Geometry: final body of the model. Coordinates: model frame, mm. Face numbers are marked on the shaded views. A direction names the side the tool comes from. Give positions to 0.01 mm unless a question says otherwise; leave off trailing zeros. Write each loop counter-clockwise with the first axis right and the second up, starting at its lowest first coordinate (ties: lowest second). Pieces come first, ordered by that corner, then holes.
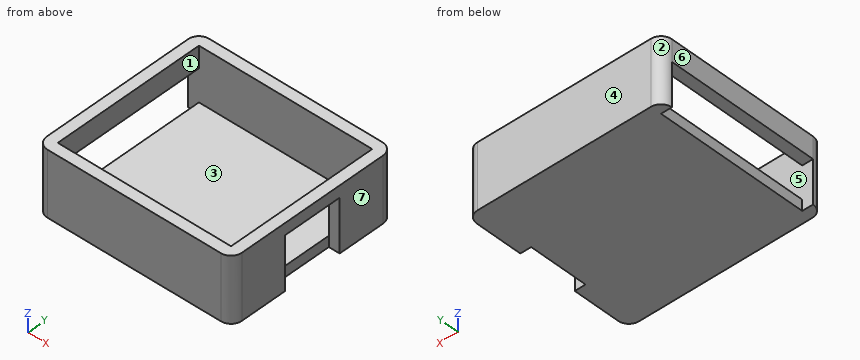
from build123d import *

# Parameters (mm, degrees)
F1_DEPTH = 19.05
F2_T     = 3.175
F3_W     = 17.145
F3_H     = 15.621
F4_DEPTH = 3.175
F5_W     = 44.45
F5_H     = 12.7
F6_DEPTH = 3.175


# Not quite as in the source:
# - a shell that OpenCascade refuses in one call is made with other operations: the cavity is built on its own and cut out


with BuildPart() as f1:
    # F0 (on Top) → F1 (new body)
    with BuildSketch(Plane.XY):
        with BuildLine():
            Line((-25.4, -25.4), (25.4, -25.4))
            ThreePointArc((25.4, -25.4), (27.6450640303, -24.4700640303), (28.575, -22.225))
            Line((28.575, -22.225), (28.575, 22.225))
            ThreePointArc((28.575, 22.225), (27.6450640303, 24.4700640303), (25.4, 25.4))
            Line((25.4, 25.4), (-25.4, 25.4))
            ThreePointArc((-25.4, 25.4), (-27.6450640303, 24.4700640303), (-28.575, 22.225))
            Line((-28.575, 22.225), (-28.575, -22.225))
            ThreePointArc((-28.575, -22.225), (-27.6450640303, -24.4700640303), (-25.4, -25.4))
        make_face()
    extrude(amount=F1_DEPTH)

    # F2: shell of thickness 3.175, made by hand


with BuildPart() as f2_core1:
    # F2_t2: copy of F1
    add(f1.part)

    # the walls: a layer under each face that stays
    f2_faces = [f2_core1.faces().sort_by_distance(p)[0] for p in [
        (0, -25.4, 9.525),
        (28.575, 0, 9.525),
        (0, 25.4, 9.525),
        (-28.575, 0, 9.525),
        (0, 0, 0),
    ]]
    thicken(f2_faces, amount=-F2_T, mode=Mode.SUBTRACT)


with BuildPart() as f1_1:
    add(f1.part)

    # what is left inside the walls is the cavity
    f2_cavity = [f2_core1.part.solids().sort_by_distance(p)[0] for p in [
        (0, -7.408333, 3.20675),
    ]]
    add(f2_cavity, mode=Mode.SUBTRACT)

    # F3 (on face) → F4 (cut)
    with BuildSketch(Plane.YZ.offset(28.575)):
        with Locations((0, 7.8105)):
            Rectangle(F3_W, F3_H)
    extrude(amount=-F4_DEPTH, mode=Mode.SUBTRACT)

    # F5 (on face) → F6 (cut)
    with BuildSketch(Plane(origin=(-28.575, 0, 0), x_dir=(0, -1, 0), z_dir=(-1, 0, 0))):
        with Locations((0, 6.35)):
            Rectangle(F5_W, F5_H)
    extrude(amount=-F6_DEPTH, mode=Mode.SUBTRACT)


solid = f1_1.part
Q1. Section D-D on x = -4. Output: boundary loops of the cut face in (y, z) (3 decimals).
Filled sheet:
outline: (-25.4, 0) - (25.4, 0) - (25.4, 19.05) - (22.225, 19.05) - (22.225, 3.175) - (-22.225, 3.175) - (-22.225, 19.05) - (-25.4, 19.05) - close
Q2. Section B-B on z = 16.5. Output: boundary loops of the cut face in (x, y) (3 decimals).
Filled sheet:
outline: (-28.575, -22.225) arc R3.175 ccw to (-25.4, -25.4) - (25.4, -25.4) arc R3.175 ccw to (28.575, -22.225) - (28.575, 22.225) arc R3.175 ccw to (25.4, 25.4) - (-25.4, 25.4) arc R3.175 ccw to (-28.575, 22.225) - close; hole (-25.4, -22.225) - (25.4, -22.225) - (25.4, 22.225) - (-25.4, 22.225) - close
Q3. Pin query (flat end, axial travel): P1, Ø1.6, axis at x = 27, y = -2.5, coming from the -Z side; P2, Ø1.6, axis at x = 27.5, z = 7.5, coming from the -Y side; P3, Ø1, axis at y = 8, z = 12.5, coming from the +X side; P4, Ø8, axis at y = -0.5, z = 10, coming from the -X side (3 decimals). Return the tip coordinate at first contact, or that it passes through.
Filled sheet:
P1: stops at z = 15.62
P2: stops at y = -25.12
P3: stops at x = -25.4
P4: stops at x = -28.575
Q4. Access query for the marked faces 1, 2 and 3. Directions: +Z, -Z, +X, -X, +Y, -Y. A direction counts if a zero-diameter tool reaches every point of the face in a straight line with its end or side. Return the directions, or none.
Filled sheet:
face 1: +Z
face 2: +Z, -Z, -X, +Y
face 3: +Z, -X
Q5. Section A-A on y = 13.5. Output: boundary loops of the cut face in (x, z) (3 decimals), plus the area to 3 significant figures.
Filled sheet:
outline: (-28.575, 12.7) - (-25.4, 12.7) - (-25.4, 19.05) - (-28.575, 19.05) - close; (-25.4, 0) - (28.575, 0) - (28.575, 19.05) - (25.4, 19.05) - (25.4, 3.175) - (-25.4, 3.175) - close
area: 242 mm2
Q6. Ray query, line 1 along Y through (x, z) = (14.5, 10.5) (3 decimals); line 2 along X through (y, z) = (21, 16) (3 decimals); line 3 along X through (y, z) = (6, 1.75). Return the intervals inside material, ascending.
Filled sheet:
line 1: y = -25.4 to -22.225, 22.225 to 25.4
line 2: x = -28.575 to -25.4, 25.4 to 28.575
line 3: x = -25.4 to 25.4
Q7. Pull-direction query (X, two-part tool) for the marked faces 4, 5, 6 and 7; classes: released by +X, released by -X, zero draft, split by the parting line, or undercut.
Filled sheet:
face 4: zero draft
face 5: undercut
face 6: released by -X
face 7: released by +X
